```python
from build123d import *

# Parameters (mm, degrees)
SZKIC1_W                    = 170
SZKIC1_H                    = 50
DODANIE_WYCI_GNI_CIE1_DEPTH = 5
SZKIC2_W                    = 0.7
SZKIC2_H                    = 31
WYTNIJ_WYCI_GNI_CIE1_DEPTH  = 173.234529168
SZKIC3_W                    = 1
SZKIC3_H                    = 26
WYTNIJ_WYCI_GNI_CIE2_DEPTH  = 173.234529168
SZKIC4_R                    = 1.7
WYTNIJ_WYCI_GNI_CIE3_DEPTH  = 101.51922361
SZKIC5_R                    = 22.5
WYTNIJ_WYCI_GNI_CIE4_DEPTH  = 10
WYTNIJ_WYCI_GNI_CIE5_DEPTH  = 101.51922361
LUSTRO2_COPY_1_DEPTH        = 101.51922361
SZKIC7_W                    = 32.832404509
SZKIC7_H                    = 9.5
DODANIE_WYCI_GNI_CIE2_DEPTH = 5
SZKIC8_W                    = 34.236470266
SZKIC8_H                    = 9.5
DODANIE_WYCI_GNI_CIE3_DEPTH = 5
SZKIC9_W                    = 39.464340028
SZKIC9_H                    = 2.5
DODANIE_WYCI_GNI_CIE4_DEPTH = 4.3
SZKIC10_W                   = 39.512976603
SZKIC10_H                   = 2.5
DODANIE_WYCI_GNI_CIE5_DEPTH = 4.3


with BuildPart() as part:
    # Szkic1 → Dodanie-wyciągnięcie1 (new body)
    with BuildSketch(Plane.XY):
        with Locations((11.640474324, -2.198033708)):
            Rectangle(SZKIC1_W, SZKIC1_H)
    extrude(amount=DODANIE_WYCI_GNI_CIE1_DEPTH)

    # Szkic2 → Wytnij-wyciągnięcie1 (cut, through all)
    with BuildSketch(Plane.ZY.offset(73.359525676)):
        with Locations((0.35, -2.198033708)):
            Rectangle(SZKIC2_W, SZKIC2_H)
    extrude(amount=-WYTNIJ_WYCI_GNI_CIE1_DEPTH, mode=Mode.SUBTRACT)

    # Szkic3 → Wytnij-wyciągnięcie2 (cut, through all)
    with BuildSketch(Plane.ZY.offset(73.359525676)):
        with Locations((1.2, -2.198033708)):
            Rectangle(SZKIC3_W, SZKIC3_H)
    extrude(amount=-WYTNIJ_WYCI_GNI_CIE2_DEPTH, mode=Mode.SUBTRACT)

    # Szkic4 → Wytnij-wyciągnięcie3 (cut, through all)
    with BuildSketch(Plane.XY.offset(5)):
        with Locations((-8.359525676, -22.198033708)):
            Circle(SZKIC4_R)
        with Locations((31.640474324, -22.198033708)):
            Circle(SZKIC4_R)
        with Locations((31.640474324, 17.801966292)):
            Circle(SZKIC4_R)
        with Locations((-8.359525676, 17.801966292)):
            Circle(SZKIC4_R)
    extrude(amount=-WYTNIJ_WYCI_GNI_CIE3_DEPTH, mode=Mode.SUBTRACT)

    # Szkic5 → Wytnij-wyciągnięcie4 (cut)
    with BuildSketch(Plane.XY.offset(5)):
        with Locations((11.640474324, -2.198033708)):
            Circle(SZKIC5_R)
    extrude(amount=-WYTNIJ_WYCI_GNI_CIE4_DEPTH, mode=Mode.SUBTRACT)

    # Szkic6 → Wytnij-wyciągnięcie5 (cut, through all)
    with BuildSketch(Plane(origin=(0, 0, 0), x_dir=(-1, 0, 0), z_dir=(0, 0, -1))):
        with BuildLine():
            Line((66.359525676, 19.751966292), (61.359525676, 19.751966292))
            ThreePointArc((61.359525676, 19.751966292), (59.659525676, 18.051966292), (61.359525676, 16.351966292))
            Line((61.359525676, 16.351966292), (66.359525676, 16.351966292))
            ThreePointArc((66.359525676, 16.351966292), (68.059525676, 18.051966292), (66.359525676, 19.751966292))
        make_face()
    wytnij_wyci_gni_cie5 = extrude(amount=-WYTNIJ_WYCI_GNI_CIE5_DEPTH, mode=Mode.SUBTRACT)

    # Lustro1: Wytnij-wyciągnięcie5 across plane
    add(wytnij_wyci_gni_cie5.mirror(Plane(origin=(0, -2.198033708, 0), x_dir=(0, 0, 1), z_dir=(0, -1, 0))), mode=Mode.SUBTRACT)

    # Lustro2: Wytnij-wyciągnięcie5 across plane
    add(wytnij_wyci_gni_cie5.mirror(Plane(origin=(11.640474324, 0, 0), x_dir=(0, 0, 1), z_dir=(1, 0, 0))), mode=Mode.SUBTRACT)

    # Lustro2 copy 1 sketch → Lustro2 copy 1 (cut, through all)
    with BuildSketch(Plane(origin=(23.280948648, -4.396067416, 0), x_dir=(1, 0, 0), z_dir=(0, 0, -1))):
        with BuildLine():
            Line((66.359525676, 19.751966292), (61.359525676, 19.751966292))
            ThreePointArc((61.359525676, 19.751966292), (59.659525676, 18.051966292), (61.359525676, 16.351966292))
            Line((61.359525676, 16.351966292), (66.359525676, 16.351966292))
            ThreePointArc((66.359525676, 16.351966292), (68.059525676, 18.051966292), (66.359525676, 19.751966292))
        make_face()
    extrude(amount=-LUSTRO2_COPY_1_DEPTH, mode=Mode.SUBTRACT)

    # Szkic7 → Dodanie-wyciągnięcie2 (add, through all)
    with BuildSketch(Plane(origin=(0, 0, 0), x_dir=(-1, 0, 0), z_dir=(0, 0, -1))):
        with Locations((-11.5337785, 18.051966292)):
            Rectangle(SZKIC7_W, SZKIC7_H)
    extrude(amount=-DODANIE_WYCI_GNI_CIE2_DEPTH)

    # Szkic8 → Dodanie-wyciągnięcie3 (add, through all)
    with BuildSketch(Plane(origin=(0, 0, 0), x_dir=(-1, 0, 0), z_dir=(0, 0, -1))):
        with Locations((-10.831745621, -22.448033708)):
            Rectangle(SZKIC8_W, SZKIC8_H)
    extrude(amount=-DODANIE_WYCI_GNI_CIE3_DEPTH)

    # Szkic9 → Dodanie-wyciągnięcie4 (add, through all)
    with BuildSketch(Plane(origin=(0, 0, 0.7), x_dir=(-1, 0, 0), z_dir=(0, 0, -1))):
        with Locations((-10.272671982, 12.051966292)):
            Rectangle(SZKIC9_W, SZKIC9_H)
    extrude(amount=-DODANIE_WYCI_GNI_CIE4_DEPTH)

    # Szkic10 → Dodanie-wyciągnięcie5 (add, through all)
    with BuildSketch(Plane(origin=(0, 0, 0.7), x_dir=(-1, 0, 0), z_dir=(0, 0, -1))):
        with Locations((-10.248353695, -16.448033708)):
            Rectangle(SZKIC10_W, SZKIC10_H)
    extrude(amount=-DODANIE_WYCI_GNI_CIE5_DEPTH)


solid = part.part
```
Here's how the part is built. I have some questions about the finished solid (model axes, mm). A direction names the side the tool comes from. Coordinates: 2 decimals unless noted, no trailing zeros. Order: outer loops, then holes, each group sorted by start corner. A loop starts at its lowest first (then second) coordinate and runs counter-clockwise, first axis right, second up.
1) Will these pins go through, and if not, where does the flat tip stop? pin 1 (4.5 mm diameter, centred on x = -8.36, y = 17.8, fed in from +Z); pin 2 (8 mm diameter, centred on x = 79, y = 4, fed in from -Z); pin 3 (2 mm diameter, centred on x = 10, y = 11.5, fed in from -Z).
2) Imagine slicing it at A-A on x = 2. List the corners of the cut face in (y, z) for me, and give its area (4 significant figures).
3) Imagine slicing it at D-D on z = 3.9. State how many separate pieces and enclosed holes the cut face has, and give its area (3 significant figures).
4) Imagine slicing it at C-C on x = -23. List the corners of the cut face in (y, z) for me, and give its area (3 significant figures).
5) Imagine slicing it at B-B on y = 0.5. List the corners of the cut face in (x, z) for me, and give its area (3 significant figures).
6) We'd pull the mould along Y, two halves only. Please class faces 5 (the face through (34.14, -2.39, 3.37)), 6 (the face through (13, 15, 5)), 7 (the face through (13, -27.198, 2)): +Y half, -Y half, draft (parallel to the pull), parting line (faces both ways), or undercut.
7) I need wall thicknesses on line 1 (X direction, y = 18, z = 0.75); line 2 (Y direction, x = -40, z = 0.9); line 3 (X direction, y = 17.5, z = 1.35). Which ranges of each line are inside material? Lowest first, please.
8) Which directions (+Z, -Z, +X, -X, +Y, -Y) give clear straight access to the entire face, cutting with the end or side of a thin tool? Please do faces 1 (the face through (-73.36, -3, 3)), 2 (the face through (63, -2, 1.7)), 3 (the face through (13, -15.198, 2)), 4 (the face through (-64, 16.352, 2)).
Response values:
1. pin 1: stops at z = 5
1. pin 2: stops at z = 1.7
1. pin 3: stops at z = 0.7
2. outline: (-27.2, 0) - (-17.7, 0) - (-17.7, 0.7) - (-15.2, 0.7) - (-15.2, 5) - (-27.2, 5) - close; (10.8, 0.7) - (13.3, 0.7) - (13.3, 0) - (22.8, 0) - (22.8, 5) - (10.8, 5) - close
2. area: 116.5 mm2
3. separate pieces: 1
3. enclosed holes: 9
3. area: 7,260 mm2
4. outline: (-27.2, 0) - (-17.7, 0) - (-17.7, 0.7) - (-15.2, 0.7) - (-15.2, 1.7) - (10.8, 1.7) - (10.8, 0.7) - (13.3, 0.7) - (13.3, 0) - (22.8, 0) - (22.8, 5) - (-27.2, 5) - close
4. area: 202 mm2
5. outline: (-73.36, 1.7) - (-10.7, 1.7) - (-10.7, 5) - (-73.36, 5) - close; (33.98, 1.7) - (96.64, 1.7) - (96.64, 5) - (33.98, 5) - close
5. area: 414 mm2
6. face 5: undercut
6. face 6: draft
6. face 7: -Y half
7. line 1: x = -73.36 to -68.06, -59.66 to -10.05, -6.67 to 29.95, 33.33 to 82.94, 91.34 to 96.64
7. line 2: y = -27.2 to -15.2, 10.8 to 22.8
7. line 3: x = -73.36 to -67.97, -59.75 to -10.03, -6.69 to 29.97, 33.31 to 83.03, 91.25 to 96.64
8. face 1: +Z, -Z, -X, +Y, -Y
8. face 2: -Z, +X, -X
8. face 3: -Z
8. face 4: +Z, -Z
